from build123d import *

# Parameters (mm, degrees)
SKETCH1_W           = 8.177357898
SKETCH1_H           = 5.946767651
BOSS_EXTRUDE1_DEPTH = 15
SKETCH2_R           = 1.27


with BuildPart() as part:
    # Sketch1 → Boss-Extrude1 (new body)
    with BuildSketch(Plane.XY):
        with Locations((-51.319507827, 71.357432061)):
            Rectangle(SKETCH1_W, SKETCH1_H)
    extrude(amount=-BOSS_EXTRUDE1_DEPTH)

    # Sweep1: sweep along a path in Sketch3
    with BuildLine(Plane.XY.offset(-9.522776034)) as sweep1_path:
        Line((-51.319507827, 68.384048236), (-51.319507827, -20.048994445))
        ThreePointArc((-51.319507827, -20.048994445), (-39.023171295, -32.345330977), (-26.726834763, -20.048994445))
        Line((-26.726834763, -20.048994445), (-26.726834763, 48.210546245))
        ThreePointArc((-26.726834763, 48.210546245), (-13.409077555, 61.528303453), (-0.091320347, 48.210546245))
        Line((-0.091320347, 48.210546245), (-0.091320347, -27.444646548))
    # Sketch2 → Sweep1 (sweep)
    with BuildSketch(Plane.XZ.offset(-68.384048236)):
        with Locations((-51.319507827, -9.522776034)):
            Circle(SKETCH2_R)
    sweep(path=sweep1_path.line)


solid = part.part
Could you check a few things on this model? Use its own coordinates, in mm. A direction names the side the tool comes from. Give positions to 0.01 mm unless a question says otherwise; leave off trailing zeros. Write each loop counter-clockwise with the first axis right and the second up, starting at its lowest first coordinate (ties: lowest second). Pieces come first, ordered by that corner, then holes. Notation, with made-up numbers: (-33.75, 75.5) -> (-15.75, 75.5) arc R3 cw to (-15.75, 79.5) -> close; hole circle Ø8 at (50, 63). An arc over 180 degrees is marked (long way). Answer as CSV lines item,"result". Start each with the question number.
(1) If we section it at A-A, the plane y = 13: Write out the boundary of the cut face in (x, z), and give its area (3 significant figures).
(2) Which directions (+Z, -Z, +X, -X, +Y, -Y) give clear straight access to the entire face, cutting with the end or side of a thin tool? Please do faces 4 (the face through (0, -27.445, -10)), 5 (the face through (-47.231, 71, -7)), 6 (the face through (-27.938, 14.559, -9.141)).
(3) If we section it at C-C, the plane y = -25.5: Give the number of separate pieces and of enclosed holes in the cut face, and give its area (3 significant figures).
(4) If we section it at B-B, the plane z = -2.75: Write out the boundary of the cut face in (x, y).
(5) I'm going to push flat-ended pins straight in: pin 1 Ø5 at (y, z) = (70.5, -10) entering from +X; pin 2 Ø3 at (x, z) = (0, -10) entering from -Y; pin 3 Ø1 at (x, z) = (-9, -10.5) entering from +Y. Where does each tip first touch, or does it pass through?
(6) Please list where these lines run through material, in increasing order: line 1 (X direction, y = 32.5, z = -9.5); line 2 (X direction, y = -9, z = -10.25); line 3 (Y direction, x = -49.5, z = -6.5).
(7) If we mould it in two halves opening along X, with no side actions, what happens to faces 1 (the face through (-55.408, 71, -7)), 2 (the face through (-51, 74.331, -7)), 3 (the face through (-52.59, 23.55, -9.47))? For each: +X half, -X half, draft (parallel to the pull), parting line (faces both ways), or undercut.
Answer list:
1,outline,"circle Ø2.54 at (-51.32, -9.52); circle Ø2.54 at (-26.73, -9.52); circle Ø2.54 at (-0.09, -9.52)"
1,area,"15.2 mm^2"
2,face 4,"+Z, -Z, +X, -Y"
2,face 5,"+Z, -Z, +X, +Y"
2,face 6,"none"
3,separate pieces,"3"
3,enclosed holes,"0"
3,area,"16.4 mm^2"
4,outline,"(-55.41, 68.38) -> (-47.23, 68.38) -> (-47.23, 74.33) -> (-55.41, 74.33) -> close"
5,pin 1,"x = -47.23"
5,pin 2,"y = -27.44"
5,pin 3,"y = 62.07"
6,line 1,"-52.59 to -50.05, -28 to -25.46, -1.36 to 1.18"
6,line 2,"-52.36 to -50.28, -27.77 to -25.69, -1.13 to 0.95"
6,line 3,"68.38 to 74.33"
7,face 1,"-X half"
7,face 2,"draft"
7,face 3,"undercut"
